Verification items for the finished model (mm, model axes). Face numbers are marked on the shaded views. Give positions to 0.01 mm unless a question says otherwise; leave off trailing zeros. Loops run counter-clockwise (first coordinate to the right, second up) from the corner with the lowest first, then second, coordinate; pieces in that order, holes last. Notation, with made-up numbers: (-25.5, 7) - (7.5, 7) arc R16 ccw to (7.5, 13) - close; hole circle Ø2 at (-3, -13.5). An arc over 180 degrees is marked (long way). One line per question, with ' | ' between items. Start each with the question number.
1. Mould release check, pull along X, two halves, no side actions. Record for the marked faces 1, 2 and 3: +X half, -X half, draft (parallel to the pull), parting line (faces both ways), or undercut.
2. Section check C-C, the plane z = 3.75. Enter the section's corners in (x, y), then the cut area to 3 significant figures.
3. Thickness scan on line 1 along Y through (x, z) = (0, 8.75); line 2 along X through (y, z) = (1, 8.25); line 3 along X through (y, z) = (1.75, 3.5). Record the ranges inside material, lowest first. Write a range as from..to.
4. Depth check by flat-ended pin: pin 1 Ø3 at (x, z) = (-2, 2.5) entering from +Y; pin 2 Ø4 at (y, z) = (-2.5, 3) entering from -X; pin 3 Ø3 at (y, z) = (3, 5) entering from +X. Enter the tip coordinate at first touch or a pass-through.
5. Section check A-A, the plane x = 0. Enter the section's corners in (y, z).
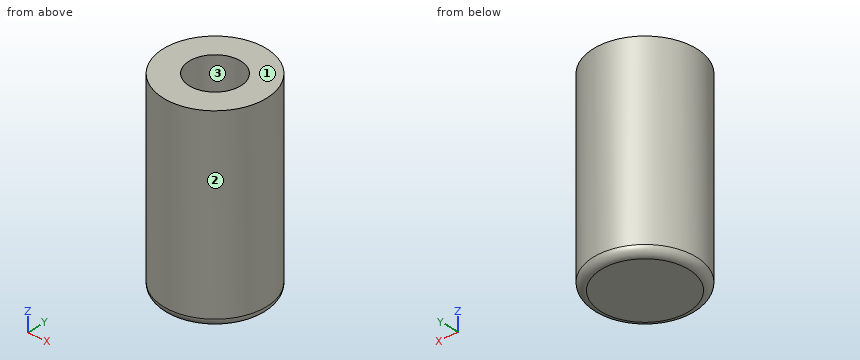
from build123d import *

# Parameters (mm, degrees)
SKETCH1_R           = 4
BOSS_EXTRUDE1_DEPTH = 15
SKETCH2_R           = 2
CUT_EXTRUDE1_DEPTH  = 13
FILLET1_R           = 0.6


with BuildPart() as part:
    # Sketch1 → Boss-Extrude1 (new body)
    with BuildSketch(Plane.XY):
        Circle(SKETCH1_R)
    extrude(amount=BOSS_EXTRUDE1_DEPTH)

    # Sketch2 → Cut-Extrude1 (cut)
    with BuildSketch(Plane.XY.offset(15)):
        Circle(SKETCH2_R)
    extrude(amount=-CUT_EXTRUDE1_DEPTH, mode=Mode.SUBTRACT)

    # Fillet1
    fillet1_edges = [part.edges().sort_by_distance(p)[0] for p in [
        (-4, 0, 0),
    ]]
    fillet(fillet1_edges, radius=FILLET1_R)


solid = part.part
Results list:
1) face 1: draft | face 2: parting line | face 3: undercut
2) outline: circle Ø8 at (0, 0); hole circle Ø4 at (0, 0) | area: 37.7 mm²
3) line 1: -4..-2, 2..4 | line 2: -3.87..-1.73, 1.73..3.87 | line 3: -3.6..-0.97, 0.97..3.6
4) pin 1: y = 3.97 | pin 2: x = -3.97 | pin 3: x = 3.71
5) outline: (-4, 0.6) arc R0.6 ccw to (-3.4, 0) - (3.4, 0) arc R0.6 ccw to (4, 0.6) - (4, 15) - (2, 15) - (2, 2) - (-2, 2) - (-2, 15) - (-4, 15) - close
